from build123d import *

# Parameters (mm, degrees)
SKETCH_1_W               = 50
SKETCH_1_H               = 20
EXTRUDE_1_DEPTH          = 10
CUT_EXTRUDE_1_DEPTH      = 57
CUT_EXTRUDE_2_DEPTH      = 57
EXTRUDE_2_DEPTH          = 20
EXTRUDE_3_DEPTH          = 20
CUT_EXTRUDE_3_DEPTH      = 3
CUT_EXTRUDE_3_DEPTH_BACK = 16
SKETCH_7_R               = 1.5
SKETCH_12_R              = 1.6
CUT_EXTRUDE_4_DEPTH      = 13
SKETCH_13_R              = 5.5
CUT_EXTRUDE_6_DEPTH      = 1.7


with BuildPart() as part:
    # 草图1 → 凸台-拉伸1 (new body)
    with BuildSketch(Plane(origin=(0, 0, 0), x_dir=(1, 0, 0), z_dir=(0, 1, 0))):
        Rectangle(SKETCH_1_W, SKETCH_1_H)
    extrude(amount=EXTRUDE_1_DEPTH)

    # 草图2 → 切除-拉伸1 (cut)
    with BuildSketch(Plane.ZY.offset(25)):
        Polygon((7, 4), (-7, 4), (-5, 9), (5, 9), align=None)
    extrude(amount=-CUT_EXTRUDE_1_DEPTH, mode=Mode.SUBTRACT)

    # 草图3 → 切除-拉伸2 (cut)
    with BuildSketch(Plane.ZY.offset(25)):
        Polygon((-5, 9), (-5, 16.661524688), (-5, 24.510715087), (5, 24.510715087), (5, 9), align=None)
    extrude(amount=-CUT_EXTRUDE_2_DEPTH, mode=Mode.SUBTRACT)

    # 草图5 → 凸台-拉伸2 (add)
    with BuildSketch(Plane.XY.offset(10)):
        with BuildLine():
            Line((-25, 0), (-25, 30))
            add(Edge.make_bspline(
                [(-25, 30), (-34.394309347, 16.149944275), (-33.463121006, 0)],
                knots=[0, 0, 0, 1, 1, 1], degree=2))
            Line((-33.463121006, 0), (-25, 0))
        make_face()
    extrude(amount=-EXTRUDE_2_DEPTH)

    # 草图6 → 凸台-拉伸3 (add)
    with BuildSketch(Plane(origin=(0, 0, -10), x_dir=(-1, 0, 0), z_dir=(0, 0, -1))):
        with BuildLine():
            Line((25, 11.927521415), (25, 10))
            add(Edge.make_bspline(
                [(25, 10), (24.19442895, 10.965387518), (25, 11.927521415)],
                knots=[0, 0, 0, 1, 1, 1], degree=2))
        make_face()
        with BuildLine():
            Line((25, 14.927521415), (25, 13))
            add(Edge.make_bspline(
                [(25, 13), (24.19442895, 13.965387518), (25, 14.927521415)],
                knots=[0, 0, 0, 1, 1, 1], degree=2))
        make_face()
        with BuildLine():
            Line((25, 17.927521415), (25, 16))
            add(Edge.make_bspline(
                [(25, 16), (24.19442895, 16.965387518), (25, 17.927521415)],
                knots=[0, 0, 0, 1, 1, 1], degree=2))
        make_face()
        with BuildLine():
            Line((25, 20.927521415), (25, 19))
            add(Edge.make_bspline(
                [(25, 19), (24.19442895, 19.965387518), (25, 20.927521415)],
                knots=[0, 0, 0, 1, 1, 1], degree=2))
        make_face()
        with BuildLine():
            Line((25, 23.927521415), (25, 22))
            add(Edge.make_bspline(
                [(25, 22), (24.19442895, 22.965387518), (25, 23.927521415)],
                knots=[0, 0, 0, 1, 1, 1], degree=2))
        make_face()
        with BuildLine():
            Line((25, 26.927521415), (25, 25))
            add(Edge.make_bspline(
                [(25, 25), (24.19442895, 25.965387518), (25, 26.927521415)],
                knots=[0, 0, 0, 1, 1, 1], degree=2))
        make_face()
        with BuildLine():
            Line((25, 29.927521415), (25, 28))
            add(Edge.make_bspline(
                [(25, 28), (24.19442895, 28.965387518), (25, 29.927521415)],
                knots=[0, 0, 0, 1, 1, 1], degree=2))
        make_face()
    extrude(amount=-EXTRUDE_3_DEPTH)

    # 草图7 → 切除-拉伸3 (cut, two sides: drawn at the far end of the back side and taken through both)
    with BuildSketch(Plane(origin=(-25, 0, 0), x_dir=(0, 0, -1), z_dir=(1, 0, 0)).offset(-CUT_EXTRUDE_3_DEPTH_BACK)):
        with Locations(Location((0, 7, 0), (0, 0, 180))):
            Circle(SKETCH_7_R)
    extrude(amount=CUT_EXTRUDE_3_DEPTH + CUT_EXTRUDE_3_DEPTH_BACK, mode=Mode.SUBTRACT)

    # 草图12 → 切除-拉伸4 (cut)
    with BuildSketch(Plane.XZ):
        with Locations(Location((-4.231560503, 3, 0), (0, 0, 270))):
            Circle(SKETCH_12_R)
        with Locations(Location((-4.231560503, -3, 0), (0, 0, 270))):
            Circle(SKETCH_12_R)
        with Locations(Location((-1.231560503, 0, 0), (0, 0, 270))):
            Circle(SKETCH_12_R)
        with Locations(Location((-7.231560503, 0, 0), (0, 0, 270))):
            Circle(SKETCH_12_R)
    extrude(amount=-CUT_EXTRUDE_4_DEPTH, mode=Mode.SUBTRACT)

    # 草图13 → 切除-拉伸6 (cut)
    with BuildSketch(Plane(origin=(0, 4, 0), x_dir=(1, 0, 0), z_dir=(0, 1, 0))):
        with Locations(Location((-4.231560503, 0, 0), (0, 0, 270))):
            Circle(SKETCH_13_R)
    extrude(amount=-CUT_EXTRUDE_6_DEPTH, mode=Mode.SUBTRACT)


solid = part.part
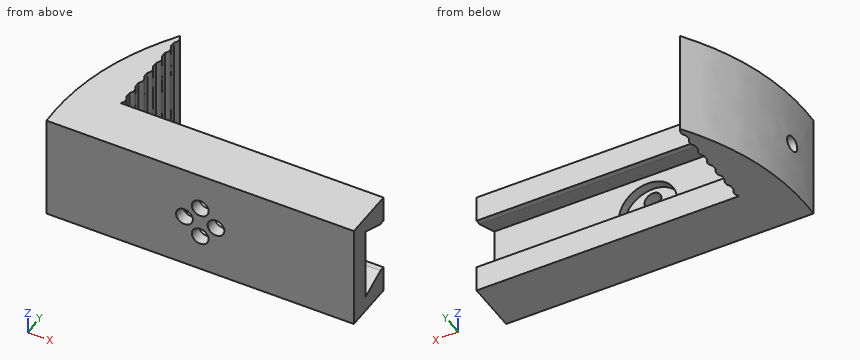
Read the model definition and answer for the solid it produces. Units are mm, in the model's axes. Round coordinates to 2 decimals unless told otherwise and drop trailing zeros. Write each loop counter-clockwise with the first axis right and the second up, starting at its lowest first coordinate (ties: lowest second). Pieces come first, ordered by that corner, then holes. Notation, with made-up numbers: (17.25, 37) - (58.25, 37) arc R16 cw to (58.25, 43) - close; hole circle Ø2 at (12, 81). An arc over 180 degrees is marked (long way). Use a Markdown table: item, result.
(1) Straight lines are drawn through the part: line 1 along Y through (x, z) = (1, 1.5); line 2 along Y through (x, z) = (1.5, -9); line 3 along X through (y, z) = (1.65, -3). For each, find the intervals that lie inside material, in ascending order. Write a range as [from, to].
Reported:
| item | result |
|---|---|
| line 1 | [0, 2.3] |
| line 2 | [0, 10] |
| line 3 | [-33.53, -5.83], [-2.63, 25] |
(2) Each of these flat-tipped pins is pushed along its axis until it touches: pin 1 Ø4 at (y, z) = (14, 6) entering from +X; pin 2 Ø0.9 at (y, z) = (15.5, 4) entering from +X; pin 3 Ø5 at (y, z) = (8, -2.5) entering from +X; pin 4 Ø3.5 at (x, z) = (-4.23, -3) entering from -Y. Where does it stop, or does it pass through?
Reported:
| item | result |
|---|---|
| pin 1 | x = -24.6 |
| pin 2 | x = -25 |
| pin 3 | x = -24.69 |
| pin 4 | y = 0 |
(3) The part is cut by section B-B (z = 0). State how many separate pieces and enclosed holes the cut face has, then the cut area to 3 significant figures.
Reported:
| item | result |
|---|---|
| separate pieces | 4 |
| enclosed holes | 0 |
| area | 327 mm2 |
(4) The part is cut by section A-A (x = 3.5). Write down the section's boundary in (y, z), then the cut area to 3 significant figures.
Reported:
| item | result |
|---|---|
| outline | (0, -10) - (10, -10) - (10, -5) - (9, -5) - (4, -7) - (4, 7) - (9, 5) - (10, 5) - (10, 10) - (0, 10) - close |
| area | 130 mm2 |
